Autodesk Fusion 360 part; units mm, degrees
sketch "Esquisse1" plane through (0, 0, 0) normal (0, 1, 0) x (1, 0, 0)
  line L0 (-305, 225) -> (305, 225)
  line L1 (325, 205) -> (325, -205)
  line L2 (305, -225) -> (223.8346, -225)
  line L3 (-325, -205) -> (-325, 205)
  line L4 (-325, 225) -> (325, -225) construction
  line L5 (325, 225) -> (-325, -225) construction
  arc A0 (209.2489, -218.6842) -> (-209.2489, -218.6842) centre (0, -415) ccw
  line L6 (-367.4671, -125) -> (350, -125) construction
  line L7 (-305, -225) -> (-223.8346, -225)
  line L8 (215, -225) -> (325, -225)
  arc A1 (209.2489, -218.6842) -> (223.8346, -225) centre (223.8346, -205) ccw
  arc A2 (305, -225) -> (325, -205) centre (305, -205) ccw
  arc A3 (325, 205) -> (305, 225) centre (305, 205) ccw
  arc A4 (-305, 225) -> (-325, 205) centre (-305, 205) ccw
  arc A5 (-325, -205) -> (-305, -225) centre (-305, -205) ccw
  arc A6 (-223.8346, -225) -> (-209.2489, -218.6842) centre (-223.8346, -205) ccw
  point P0 (-215, -225)
  dimension "d12" = 650
  dimension "d13" = 450
  dimension "d14" = 110
  dimension "d15" = 110
  dimension "d16" = 100
  dimension "d20" = 190
  dimension "d21" = 20
extrude "Extrusion1" add sketch "Esquisse1" along normal blind 4
sketch "Esquisse2" plane through (0, 4, 0) normal (0, 1, 0) x (-1, 0, 0)
  arc A0 (325, 205) -> (305, 225) centre (305, 205) ccw
  line L0 (305, 225) -> (223.8346, 225)
  arc A1 (223.8346, 225) -> (209.2489, 218.6842) centre (223.8346, 205) ccw
  arc A2 (-209.2489, 218.6842) -> (209.2489, 218.6842) centre (0, 415) ccw
  arc A3 (-209.2489, 218.6842) -> (-223.8346, 225) centre (-223.8346, 205) ccw
  line L1 (-223.8346, 225) -> (-305, 225)
  arc A4 (-305, 225) -> (-325, 205) centre (-305, 205) ccw
  line L2 (-325, 205) -> (-325, -205)
  arc A5 (-325, -205) -> (-305, -225) centre (-305, -205) ccw
  line L3 (-305, -225) -> (305, -225)
  arc A6 (305, -225) -> (325, -205) centre (305, -205) ccw
  line L4 (325, -205) -> (325, 205)
  line L5 (-50, -150) -> (50, -150)
  line L6 (50, -150) -> (50, -210)
  line L7 (50, -210) -> (-50, -210)
  line L8 (50, -210) -> (-50, -150) construction
  line L9 (-50, -210) -> (-50, -150)
  line L10 (-50, -210) -> (50, -150) construction
  point P0 (0, -275)
  point P1 (0, -180)
  dimension "d24" = 60
  dimension "d25" = 100
  dimension "d26" = 15
extrude "Extrusion2" cut sketch "Esquisse2" against normal blind 50 contours L5 L6 L7 L9
sketch "Esquisse3" plane through (0, 4, 0) normal (0, 1, 0) x (-1, 0, 0)
  line L0 (50, -150) -> (50, -210)
  line L1 (50, -210) -> (-50, -210)
  line L2 (-50, -210) -> (-50, -150)
  line L3 (-50, -150) -> (50, -150)
  arc A0 (325, 205) -> (305, 225) centre (305, 205) ccw
  line L4 (305, 225) -> (223.8346, 225)
  arc A1 (223.8346, 225) -> (209.2489, 218.6842) centre (223.8346, 205) ccw
  arc A2 (-209.2489, 218.6842) -> (209.2489, 218.6842) centre (0, 415) ccw
  arc A3 (-209.2489, 218.6842) -> (-223.8346, 225) centre (-223.8346, 205) ccw
  line L5 (-223.8346, 225) -> (-305, 225)
  arc A4 (-305, 225) -> (-325, 205) centre (-305, 205) ccw
  line L6 (-325, 205) -> (-325, -205)
  arc A5 (-325, -205) -> (-305, -225) centre (-305, -205) ccw
  line L7 (-305, -225) -> (305, -225)
  arc A6 (305, -225) -> (325, -205) centre (305, -205) ccw
  line L8 (325, -205) -> (325, 205)
  circle A7 centre (167, 75) radius 2
  circle A8 centre (243, 75) radius 2
  circle A9 centre (243, -175) radius 2
  circle A10 centre (243, -125.0704) radius 2
  circle A11 centre (167, 24.9296) radius 2
  circle A12 centre (243, 24.9296) radius 2
  circle A13 centre (167, -175) radius 2
  circle A14 centre (167, -125.0704) radius 2
  line L9 (205, -263.7962) -> (205, 261.6023) construction
  line L10 (0, -279.9296) -> (0, 210.0704) construction
  circle A15 centre (-243, 75) radius 2
  circle A16 centre (-167, -175) radius 2
  circle A17 centre (-167, -125.0704) radius 2
  circle A18 centre (-243, -125.0704) radius 2
  circle A19 centre (-243, 24.9296) radius 2
  circle A20 centre (-243, -175) radius 2
  circle A21 centre (-167, 75) radius 2
  circle A22 centre (-167, 24.9296) radius 2
  line L11 (-205, -263.7962) -> (-205, 261.6023) construction
  dimension "d29" = 4
  dimension "d30" = 38
  dimension "d31" = 4
  dimension "d32" = 38
  dimension "d33" = 205
  dimension "d34" = 50
extrude "Extrusion3" cut sketch "Esquisse3" against normal blind 25 contours A7 | A8 | A9 | A10 | A11 | A12 | A13 | A14 | A15 | A16 | A17 | A18 | A19 | A20 | A21 | A22
sketch "Esquisse4" plane through (0, 4, 0) normal (0, 1, 0) x (-1, 0, 0)
  circle A0 centre (-243, 24.9296) radius 2
  circle A1 centre (-167, -175) radius 2
  circle A2 centre (167, -175) radius 2
  circle A3 centre (167, 75) radius 2
  circle A4 centre (167, 24.9296) radius 2
  circle A5 centre (243, -125.0704) radius 2
  circle A6 centre (-167, -125.0704) radius 2
  circle A7 centre (-243, 75) radius 2
  circle A8 centre (-167, 24.9296) radius 2
  circle A9 centre (-243, -175) radius 2
  circle A10 centre (243, -175) radius 2
  circle A11 centre (243, 75) radius 2
  circle A12 centre (243, 24.9296) radius 2
  circle A13 centre (167, -125.0704) radius 2
  circle A14 centre (-243, -125.0704) radius 2
  circle A15 centre (-167, 75) radius 2
  line L0 (50, -150) -> (50, -210)
  line L1 (50, -210) -> (-50, -210)
  line L2 (-50, -210) -> (-50, -150)
  line L3 (-50, -150) -> (50, -150)
  arc A16 (325, 205) -> (305, 225) centre (305, 205) ccw
  line L4 (305, 225) -> (223.8346, 225)
  arc A17 (223.8346, 225) -> (209.2489, 218.6842) centre (223.8346, 205) ccw
  arc A18 (-209.2489, 218.6842) -> (209.2489, 218.6842) centre (0, 415) ccw
  arc A19 (-209.2489, 218.6842) -> (-223.8346, 225) centre (-223.8346, 205) ccw
  line L5 (-223.8346, 225) -> (-305, 225)
  arc A20 (-305, 225) -> (-325, 205) centre (-305, 205) ccw
  line L6 (-325, 205) -> (-325, -205)
  arc A21 (-325, -205) -> (-305, -225) centre (-305, -205) ccw
  line L7 (-305, -225) -> (305, -225)
  arc A22 (305, -225) -> (325, -205) centre (305, -205) ccw
  line L8 (325, -205) -> (325, 205)
  line L9 (305, 220) -> (223.8346, 220)
  arc A23 (223.8346, 220) -> (212.8953, 215.2631) centre (223.8346, 205) ccw
  arc A24 (-212.8953, 215.2631) -> (212.8953, 215.2631) centre (0, 415) ccw
  arc A25 (-212.8953, 215.2631) -> (-223.8346, 220) centre (-223.8346, 205) ccw
  line L10 (-223.8346, 220) -> (-305, 220)
  arc A26 (-305, 220) -> (-320, 205) centre (-305, 205) ccw
  line L11 (-320, 205) -> (-320, -205)
  arc A27 (-320, -205) -> (-305, -220) centre (-305, -205) ccw
  line L12 (-305, -220) -> (305, -220)
  arc A28 (305, -220) -> (320, -205) centre (305, -205) ccw
  line L13 (320, -205) -> (320, 205)
  arc A29 (320, 205) -> (305, 220) centre (305, 205) ccw
  dimension "d37" = -5
extrude "Extrusion4" cut sketch "Esquisse4" against normal blind 50 contours A16 L4 A17 A18 A19 L5 A20 L6 A21 L7 A22 L8
Can you work these out from the model? Positions are in its coordinate system, mm. Give positions to 0.01 mm unless a question says otherwise; leave off trailing zeros. Loops run counter-clockwise (first coordinate to the right, second up) from the corner with the lowest first, then second, coordinate; pieces in that order, holes last. Notation, with made-up numbers: (-10.75, 6.5) - (8.25, 6.5) arc R13 ccw to (8.25, 13.5) - close; hole circle Ø7 at (-40, -19). An arc over 180 degrees is marked (long way). One line per item, written item: value.
(1) If we section it at B-B, the plane y = 1.25: State how many separate pieces and enclosed holes the cut face has, plus the area to 3 significant figures.
Verdict:
separate pieces: 1
enclosed holes: 17
area: 246,000 mm^2
(2) If we section it at C-C, the plane x = -126: List the corners of the cut face in (y, z) for me, plus the area to 3 significant figures.
Verdict:
outline: (0, -220) - (4, -220) - (4, 151.67) - (0, 151.67) - close
area: 1,490 mm^2
(3) If we section it at A-A, the plane x = 43: List the corners of the cut face in (y, z) for me.
Verdict:
outline: (0, -220) - (4, -220) - (4, -210) - (0, -210) - close; (0, -150) - (4, -150) - (4, 126.26) - (0, 126.26) - close
(4) If we mould it in two halves opening along X, with no side actions, what happens to faces 1 (the face through (3.34, 2.028, 123.096)), 2 (the face through (-4, 0, -3)), 3 (the face through (315.49, 2.03, 215.72))? For each: released by +X, released by -X, zero draft, split by the parting line, or undercut.
Verdict:
face 1: undercut
face 2: zero draft
face 3: released by +X
(5) I'm going to push a flat-ended pin straight in: pin 1 (3 mm diameter, centred on x = -243, z = -125.07, fed in from -Y). Where does the tip first touch, or does it pass through?
Verdict:
pin 1: through
(6) I need wall thicknesses on line 1 along Z through (x, y) = (-243, 1.9); line 2 along X through (y, z) = (2.3, -175); line 3 along X through (y, z) = (1.4, -125). Which ranges of each line are inside material? Lowest first, please.
Verdict:
line 1: -220 to -177, -173 to -127.07, -123.07 to 22.93, 26.93 to 73, 77 to 220
line 2: -320 to -245, -241 to -169, -165 to -50, 50 to 165, 169 to 241, 245 to 320
line 3: -320 to -245, -241 to -169, -165 to 165, 169 to 241, 245 to 320
